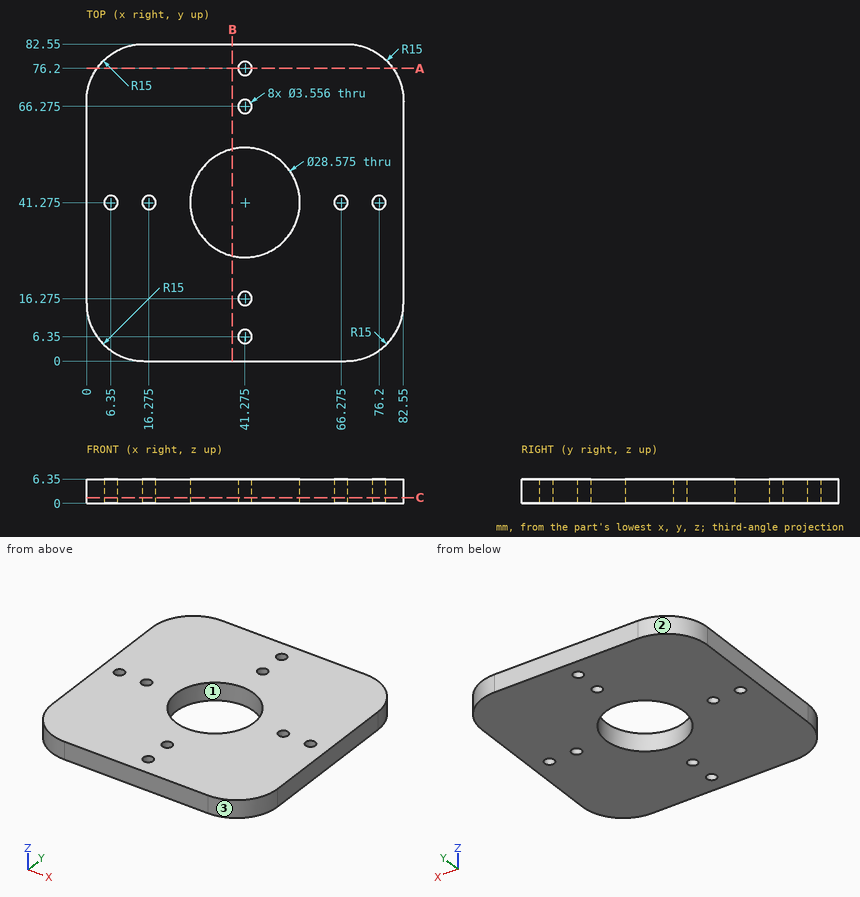
Could you check a few things on this drawing? It's one solid part, dimensions in mm from its lowest x, y, z. Round coordinates to 2 decimals unless told otherwise and drop trailing zeros. Order: outer loops, then holes, each group sorted by start corner. A loop starts at its lowest first (then second) coordinate and runs counter-clockwise, first axis right, second up. Notation, with made-up numbers: (31.25, -13.5) -> (40.25, -13.5) arc R19 ccw to (40.25, -4.5) -> close; hole circle Ø6 at (88, -10.75). An arc over 180 degrees is marked (long way). One line per question, with ' | ' between items.
Q1. If we section it at A-A on y = 76.2: Write out the boundary of the cut face in (x, z).
Computed values:
outline: (2.75, 0) -> (39.5, 0) -> (39.5, 6.35) -> (2.75, 6.35) -> close; (43.05, 0) -> (79.8, 0) -> (79.8, 6.35) -> (43.05, 6.35) -> close
Q2. If we section it at C-C on z = 1.5: Give the number of separate pieces and of enclosed holes in the cut face, plus the area to 3 significant figures.
Computed values:
separate pieces: 1 | enclosed holes: 9 | area: 5,900 mm²
Q3. If I drill on line 1 (Y direction, x = 41, z = 1); line 2 (Y direction, x = 76, z = 6); line 3 (Y direction, x = 6.35, z = 2.75), over which ranges is the centre line in solid material (lowest first)? Write a range as from..to.
Computed values:
line 1: 0..4.59, 8.11..14.52, 18.03..26.99, 55.56..64.52, 68.03..74.44, 77.96..82.55 | line 2: 2.61..39.51, 43.04..79.94 | line 3: 2.75..39.5, 43.05..79.8
Q4. We'd pull the mould along Y, two halves only. Please class the marked faces 1, 2 and 3: released by +Y, released by -Y, zero draft, split by the parting line, or undercut.
Computed values:
face 1: undercut | face 2: released by +Y | face 3: released by -Y
Q5. If we section it at B-B on x = 38: Write out the boundary of the cut face in (y, z), plus the area to 3 significant figures.
Computed values:
outline: (0, 0) -> (27.37, 0) -> (27.37, 6.35) -> (0, 6.35) -> close; (55.18, 0) -> (82.55, 0) -> (82.55, 6.35) -> (55.18, 6.35) -> close | area: 348 mm²
